Geometry check sheet. Reference: the model listing, model coordinates, mm. Coordinates: 2 decimals unless noted, no trailing zeros. Order: outer loops, then holes, each group sorted by start corner. A loop starts at its lowest first (then second) coordinate and runs counter-clockwise, first axis right, second up. Notation, with made-up numbers: (66, -39) - (88, -39) arc R17 ccw to (88, -7) - close; hole circle Ø7 at (41.5, -34.75). An arc over 180 degrees is marked (long way). Return JSON: item names as keys, results as strings. Group by question number.
Item 1: Section check B-B on z = 9. Enter the section's corners in (x, y).
Item 2: Section check D-D on x = 0.1. Enter the section's corners in (y, z) (3 decimals).
Item 3: Section check C-C on z = -6.45. Enter the section's corners in (x, y), then the cut area to 3 significant figures.
Item 4: Section check A-A on y = 0. Enter the section's corners in (x, z).
Item 5: Draft check along Y on faces 1 (the cylindrical face through (0.01, 16.84, -0.63)), 2 (the cylindrical face through (0.01, -15.13, -5.36)), 3 (the cylindrical face through (0.008, 13.343, 0.448)). Enter one of: pulls with the +Y half, pulls with the -Y half, needs draft (parallel to the pull), parting line crosses it, or undercut.
Item 6: Scan lines: probe 1 along Z at (x, y) = (-0.45, -13); probe 2 along Z at (x, y) = (-0.15, -13.5); probe 3 along Y at (x, z) = (0.25, -5.5). Record each from-to range of solid material in increasing order.
from build123d import *

# Parameters (mm, degrees)
SKETCH_1_R           = 1.25
EXTRUDE_1_DEPTH      = 0.6
EXTRUDE_1_DEPTH_BACK = 0.6


with BuildPart() as part:
    # Sketch 1 → Extrude 1 (new body, two sides)
    with BuildSketch(Plane(origin=(0, 0, 0), x_dir=(0, 0, -1), z_dir=(1, 0, 0))) as extrude_1_sk:
        with BuildLine():
            Line((-3.989591726, -13.555650403), (-3.955781017, -13.440769939))
            ThreePointArc((-3.955781017, -13.440769939), (-4.838154074, -10.666604704), (-7.741194161, -10.449963955))
            ThreePointArc((-7.741194161, -10.449963955), (-9.510855368, -10.748832352), (-11.052535247, -9.830003608))
            ThreePointArc((-11.052535247, -9.830003608), (-1.19e-07, 13.35), (11.052535397, -9.830003423))
            ThreePointArc((11.052535397, -9.830003423), (9.510855453, -10.748832336), (7.741194103, -10.449963921))
            ThreePointArc((7.741194103, -10.449963921), (4.838154048, -10.666604724), (3.955781017, -13.440769939))
            Line((3.955781017, -13.440769939), (3.989591726, -13.555650403))
            ThreePointArc((3.989591726, -13.555650403), (5.387658916, -15.140997106), (7.500750152, -15.088447473))
            ThreePointArc((7.500750152, -15.088447473), (0, 16.85), (-7.500750152, -15.088447473))
            ThreePointArc((-7.500750152, -15.088447473), (-5.387658916, -15.140997106), (-3.989591726, -13.555650403))
        make_face()
        with Locations((6.45, -12.706691151)):
            Circle(SKETCH_1_R, mode=Mode.SUBTRACT)
        with Locations((-6.45, -12.706691151)):
            Circle(SKETCH_1_R, mode=Mode.SUBTRACT)
    extrude(amount=EXTRUDE_1_DEPTH)
    extrude(extrude_1_sk.sketch, amount=-EXTRUDE_1_DEPTH_BACK)


solid = part.part
Computed:
{
 "1": {"outline": "(-0.6, -14.25) - (0.6, -14.25) - (0.6, -10.79) - (-0.6, -10.79) - close; (-0.6, 10.14) - (0.6, 10.14) - (0.6, 14.25) - (-0.6, 14.25) - close"},
 "2": {"outline": "(-15.088, -7.501) arc R16.85 ccw (long way) to (-15.088, 7.501) arc R2.5 ccw to (-13.556, 3.99) - (-13.441, 3.956) arc R2.6 ccw to (-10.45, 7.741) arc R2.6 cw to (-9.83, 11.053) arc R14.225 cw (long way) to (-9.83, -11.053) arc R2.6 cw to (-10.45, -7.741) arc R2.6 ccw to (-13.441, -3.956) - (-13.556, -3.99) arc R2.5 ccw to start; hole circle Ø2.5 at (-12.707, -6.45); hole circle Ø2.5 at (-12.707, 6.45)"},
 "3": {"outline": "(-0.6, -15.35) - (0.6, -15.35) - (0.6, -13.96) - (-0.6, -13.96) - close; (-0.6, -11.46) - (0.6, -11.46) - (0.6, -10.11) - (-0.6, -10.11) - close; (-0.6, 11.8) - (0.6, 11.8) - (0.6, 15.57) - (-0.6, 15.57) - close", "area": "7.81 mm²"},
 "4": {"outline": "(-0.6, -16.85) - (0.6, -16.85) - (0.6, -14.2) - (-0.6, -14.2) - close; (-0.6, 14.2) - (0.6, 14.2) - (0.6, 16.85) - (-0.6, 16.85) - close"},
 "5": {"face 1": "parting line crosses it", "face 2": "pulls with the -Y half", "face 3": "undercut"},
 "6": {"probe 1": "z = -10.72 to -7.67, -5.23 to -3.87, 3.87 to 5.23, 7.67 to 10.72", "probe 2": "z = -10.08 to -7.42, -5.48 to -3.97, 3.97 to 5.48, 7.42 to 10.08", "probe 3": "y = -15.19 to -13.52, -11.89 to -10.29, 12.24 to 15.93"}
}
